Geometry check sheet. Reference: the model listing, model coordinates, mm. Face numbers are marked on the shaded views. A direction names the side the tool comes from. Round coordinates to 2 decimals unless told otherwise and drop trailing zeros. Loops run counter-clockwise (first coordinate to the right, second up) from the corner with the lowest first, then second, coordinate; pieces in that order, holes last.
```python
from build123d import *

# Parameters (mm, degrees)
SKETCH_1_R      = 9.5
SKETCH_1_R_2    = 5
EXTRUDE_1_DEPTH = 1
SKETCH_2_R      = 6
SKETCH_2_R_2    = 5
EXTRUDE_2_DEPTH = 1.5
SKETCH_3_R      = 9.5
SKETCH_3_R_2    = 5
EXTRUDE_3_DEPTH = 1


with BuildPart() as part:
    # 草图1 → 凸台-拉伸1 (new body)
    with BuildSketch(Plane(origin=(0, 0, 0), x_dir=(1, 0, 0), z_dir=(0, 1, 0))):
        with Locations(Location((0, 0, 0), (0, 0, 270))):
            Circle(SKETCH_1_R)
        with Locations(Location((0, 0, 0), (0, 0, 270))):
            Circle(SKETCH_1_R_2, mode=Mode.SUBTRACT)
    extrude(amount=EXTRUDE_1_DEPTH)

    # 草图2 → 凸台-拉伸2 (add)
    with BuildSketch(Plane(origin=(0, 1, 0), x_dir=(1, 0, 0), z_dir=(0, 1, 0))):
        with Locations(Location((0, 0, 0), (0, 0, 270))):
            Circle(SKETCH_2_R)
        with Locations(Location((0, 0, 0), (0, 0, 270))):
            Circle(SKETCH_2_R_2, mode=Mode.SUBTRACT)
    extrude(amount=EXTRUDE_2_DEPTH)

    # 草图3 → 凸台-拉伸3 (add)
    with BuildSketch(Plane(origin=(0, 2.5, 0), x_dir=(1, 0, 0), z_dir=(0, 1, 0))):
        with Locations(Location((0, 0, 0), (0, 0, 270))):
            Circle(SKETCH_3_R)
        with Locations(Location((0, 0, 0), (0, 0, 270))):
            Circle(SKETCH_3_R_2, mode=Mode.SUBTRACT)
    extrude(amount=EXTRUDE_3_DEPTH)


solid = part.part
```
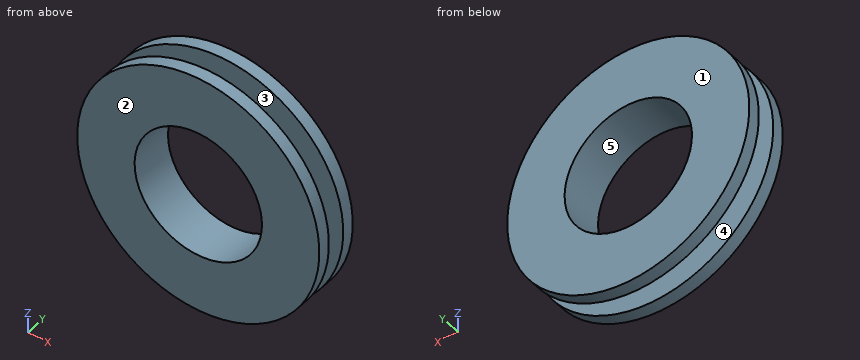
1) Gauge pin test, flat ends, axial feed: pin 1 (2 mm diameter, centred on x = -1, y = 1.5, fed in from -Z); pin 2 (1.5 mm diameter, centred on x = 5, y = 2, fed in from -Z); pin 3 (2 mm diameter, centred on x = 5, z = 2.5, fed in from -Y). Record the tip position at first contact, or that the pin passes through.
Report:
pin 1: stops at z = -9.5
pin 2: stops at z = -8.4
pin 3: stops at y = 0
2) Sectioned sample at A-A, the plane x = 0. Record the cut outline in (y, z), then the cut area to 3 significant figures.
Report:
outline: (0, -9.5) - (1, -9.5) - (1, -6) - (2.5, -6) - (2.5, -9.5) - (3.5, -9.5) - (3.5, -5) - (0, -5) - close; (0, 5) - (3.5, 5) - (3.5, 9.5) - (2.5, 9.5) - (2.5, 6) - (1, 6) - (1, 9.5) - (0, 9.5) - close
area: 21.0 mm2
3) Scan lines: line 1 along Y through (x, z) = (3.5, 7.5); line 2 along X through (y, z) = (1.15, 0); line 3 along Z through (x, y) = (-4.5, 1.35). Record each from-to range of solid material in increasing order.
Report:
line 1: y = 0 to 1, 2.5 to 3.5
line 2: x = -6 to -5, 5 to 6
line 3: z = -3.97 to -2.18, 2.18 to 3.97
4) Sectioned sample at D-D, the plane x = -7.75. Record the cut outline in (y, z), then the cut area to 3 significant figures.
Report:
outline: (0, -5.49) - (1, -5.49) - (1, 5.49) - (0, 5.49) - close; (2.5, -5.49) - (3.5, -5.49) - (3.5, 5.49) - (2.5, 5.49) - close
area: 22.0 mm2
5) Access from +Z, -Z, +X, -X, +Y, -Y to the whole of each face (thin tool, end or side, straight path). Record for the marked faces 4 and 5.
Report:
face 4: none
face 5: +Y, -Y
6) Sectioned sample at B-B, the plane z = 0. Record the cut outline in (x, y).
Report:
outline: (-9.5, 0) - (-5, 0) - (-5, 3.5) - (-9.5, 3.5) - (-9.5, 2.5) - (-6, 2.5) - (-6, 1) - (-9.5, 1) - close; (5, 0) - (9.5, 0) - (9.5, 1) - (6, 1) - (6, 2.5) - (9.5, 2.5) - (9.5, 3.5) - (5, 3.5) - close
7) Mould release check, pull along Y, two halves, no side actions. Record for the marked faces 1, 2 and 3: +Y half, -Y half, draft (parallel to the pull), parting line (faces both ways), or undercut.
Report:
face 1: +Y half
face 2: -Y half
face 3: undercut
8) Sectioned sample at C-C, the plane y = 1.75. Record the cut outline in (x, z), then the cut area to 3 significant figures.
Report:
outline: circle Ø12 at (0, 0); hole circle Ø10 at (0, 0)
area: 34.6 mm2
